Study the drawing (mm; zero at the part's minimum x, y, z) and answer. A direction names the side the tool comes from. Give positions to 0.01 mm unless a question says otherwise; leave off trailing zeros. Order: outer loops, then holes, each group sorted by start corner. A loop starts at its lowest first (then second) coordinate and runs counter-clockwise, first axis right, second up. Notation, with made-up numbers: (5.5, 70.5) - (20.5, 70.5) arc R27 cw to (20.5, 102.5) - close; hole circle Ø5 at (-15.5, 22.25). An arc over 180 degrees is marked (long way). Return JSON: item names as keys, results as strings.
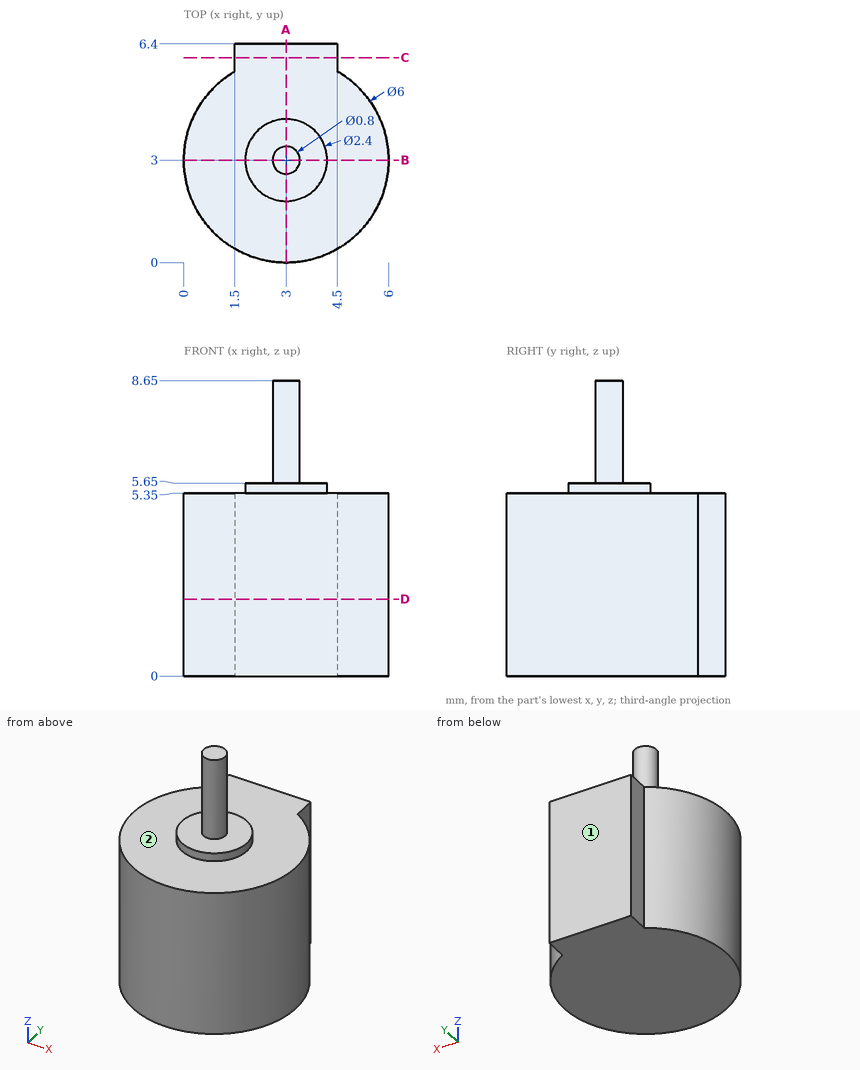
Q1. A cutting plane is placed at C-C (y = 6). Write down the section's boundary in (x, z), and give its area (4 significant figures).
Values:
{"outline": "(1.5, 0) - (4.5, 0) - (4.5, 5.35) - (1.5, 5.35) - close", "area": "16.05 mm²"}
Q2. A cutting plane is placed at B-B (y = 3). Write down the section's boundary in (x, z), and give its area (3 significant figures).
Values:
{"outline": "(0, 0) - (6, 0) - (6, 5.35) - (4.2, 5.35) - (4.2, 5.65) - (3.4, 5.65) - (3.4, 8.65) - (2.6, 8.65) - (2.6, 5.65) - (1.8, 5.65) - (1.8, 5.35) - (0, 5.35) - close", "area": "35.2 mm²"}
Q3. For the marked faces 1 and 2, determine the directions among +Z, -Z, +X, -X, +Y, -Y from which every point of the face is accessible in a straight line to the end or side of a thin tool.
Values:
{"face 1": "+Z, -Z, +X, -X, +Y", "face 2": "+Z"}
Q4. Given pin 1 (1.8 mm diameter, centred on x = 3, y = 1.5, fed in from +Z); pin 2 (0.9 mm diameter, centred on y = 6, z = 3, fed in from +X), each flat-ended and moving along its own axis, determine where each tip first touches the part or whether it passes through.
Values:
{"pin 1": "stops at z = 5.65", "pin 2": "stops at x = 4.58"}
Q5. Consider L1, parallel to Z at x = 2.75, y = 4.75; L2, parallel to X at y = 6.25, z = 2.5; L3, parallel to Y at x = 4.75, z = 4.75. Determine where each line is inside the solid, lowest interval first.
Values:
{"L1": "z = 0 to 5.35", "L2": "x = 1.5 to 4.5", "L3": "y = 0.56 to 5.44"}
Q6. A cutting plane is placed at A-A (x = 3). Write down the section's boundary in (y, z).
Values:
{"outline": "(0, 0) - (6.4, 0) - (6.4, 5.35) - (4.2, 5.35) - (4.2, 5.65) - (3.4, 5.65) - (3.4, 8.65) - (2.6, 8.65) - (2.6, 5.65) - (1.8, 5.65) - (1.8, 5.35) - (0, 5.35) - close"}
Q7. A cutting plane is placed at D-D (z = 2.25). Write down the section's boundary in (x, y), and give its area (3 significant figures).
Values:
{"outline": "(1.5, 5.6) arc R3 ccw (long way) to (4.5, 5.6) - (4.5, 6.4) - (1.5, 6.4) - close", "area": "29.9 mm²"}
